```python
from build123d import *

# Parameters (mm, degrees)
SKETCH3_R          = 14
GEARBODY_DEPTH     = 8
TOOTHCUT_DEPTH     = 22.354156504
CIRPATTERN1_COUNT  = 12
CUT_EXTRUDE1_DEPTH = 8
CHAMFER1_SIZE      = 1


with BuildPart() as part:
    # Sketch3 → gearBody (new body)
    with BuildSketch(Plane.XY):
        Circle(SKETCH3_R)
    extrude(amount=GEARBODY_DEPTH)

    # Sketch2 → toothCut (cut, through all)
    with BuildSketch(Plane.XY):
        with BuildLine():
            ThreePointArc((9.407882888, -1.636752947), (9.459378184, -1.306669437), (9.499295851, -0.974986654))
            ThreePointArc((9.499295851, -0.974986654), (9.751264317, -0.488083012), (10.267616219, -0.303844098))
            ThreePointArc((10.267616219, -0.303844098), (12.510323629, 0.19449452), (14.235972761, 1.711139825))
            ThreePointArc((14.235972761, 1.711139825), (14.203571583, -1.962007706), (13.238980983, -5.506387425))
            ThreePointArc((13.238980983, -5.506387425), (11.989111429, -3.578719403), (9.965486694, -2.491051791))
            ThreePointArc((9.965486694, -2.491051791), (9.51841766, -2.173730906), (9.407882888, -1.636752947))
        make_face()
    toothcut = extrude(amount=TOOTHCUT_DEPTH, mode=Mode.SUBTRACT)

    # CirPattern1: toothCut ×12 about axis
    cirpattern1_axis = Axis((0, 0, 0), (0, 0, 1))
    for i in range(1, CIRPATTERN1_COUNT):
        add(toothcut.rotate(cirpattern1_axis, i * 360 / CIRPATTERN1_COUNT), mode=Mode.SUBTRACT)

    # hub1Dia → Cut-Extrude1 (cut)
    with BuildSketch(Plane(origin=(0, 0, 0), x_dir=(-1, 0, 0), z_dir=(0, 0, -1))):
        with BuildLine():
            Line((-2.025, -1.590597372), (-2.025, 1.590597372))
            ThreePointArc((-2.025, 1.590597372), (2.575, 0), (-2.025, -1.590597372))
        make_face()
    extrude(amount=-CUT_EXTRUDE1_DEPTH, mode=Mode.SUBTRACT)

    # Chamfer1
    chamfer1_edges = [part.edges().sort_by_distance(p)[0] for p in [
        (-2.575, 0, 0),
        (2.025, 0, 0),
    ]]
    chamfer(chamfer1_edges, length=CHAMFER1_SIZE)


solid = part.part
```
Geometry check sheet. Reference: the model listing, model coordinates, mm. A direction names the side the tool comes from. Give positions to 0.01 mm unless a question says otherwise; leave off trailing zeros.
1. Release check for a two-part mould opening along Y. For faces 1 (the face through (2.18, 9.523, 3.944)), 2 (the face through (11.959, 2.938, 3.944)), 3 (the face through (4.445, -8.686, 3.944)) record: pulls with the +Y half, pulls with the -Y half, needs draft (parallel to the pull), parting line crosses it, or undercut.
2. Access from +Z, -Z, +X, -X, +Y, -Y to the whole of each face (thin tool, end or side, straight path). Record for faces 4 (the face through (2.025, 0, 4)), 5 (the face through (6.2, -10.58, 3.94)), 6 (the face through (-10.58, -6.2, 3.94)).
3. Gauge pin test, flat ends, axial feed: pin 1 Ø4 at (y, z) = (-1.5, 5.5) entering from +X; pin 2 Ø1.5 at (x, z) = (6.5, 5) entering from -Y; pin 3 Ø4.5 at (x, y) = (0, 0) entering from -Z (3 decimals). Record the tip position at first contact, or that the pin passes through.
4. Thickness scan on L1, parallel to Y at x = 9.75, z = 3.75; L2, parallel to X at y = -8, z = 1; L3, parallel to X at y = 0.5, z = 6.75 (3 decimals). Record the ranges inside material, lowest first.
Values follow:
1. face 1: pulls with the +Y half
1. face 2: undercut
1. face 3: pulls with the -Y half
2. face 4: +Z, -Z
2. face 5: +Z, -Z, -Y
2. face 6: +Z, -Z, -X
3. pin 1: stops at x = 13.03
3. pin 2: stops at y = -11.16
3. pin 3: stops at z = 0.775
4. L1: y = -5.87 to -2.4, -0.49 to 2.8, 5.34 to 8.75
4. L2: x = -11.39 to -7.87, -5.37 to 8.09
4. L3: x = -9.738 to -2.526, 2.025 to 13.026
